```python
from build123d import *

# Parameters (mm, degrees)
SKETCH1_R           = 125
SKETCH1_R_2         = 2.5
BOSS_EXTRUDE1_DEPTH = 4


with BuildPart() as part:
    # Sketch1 → Boss-Extrude1 (new body)
    with BuildSketch(Plane(origin=(0, 0, 0), x_dir=(1, 0, 0), z_dir=(0, 1, 0))):
        Circle(SKETCH1_R)
        with Locations((-115, 0)):
            Circle(SKETCH1_R_2, mode=Mode.SUBTRACT)
        with Locations((-99.592921435, 57.5)):
            Circle(SKETCH1_R_2, mode=Mode.SUBTRACT)
        with Locations((-57.5, 99.592921435)):
            Circle(SKETCH1_R_2, mode=Mode.SUBTRACT)
        with Locations((0, 115)):
            Circle(SKETCH1_R_2, mode=Mode.SUBTRACT)
        with Locations((57.5, 99.592921435)):
            Circle(SKETCH1_R_2, mode=Mode.SUBTRACT)
        with Locations((99.592921435, 57.5)):
            Circle(SKETCH1_R_2, mode=Mode.SUBTRACT)
        with Locations((115, 0)):
            Circle(SKETCH1_R_2, mode=Mode.SUBTRACT)
        with Locations((99.592921435, -57.5)):
            Circle(SKETCH1_R_2, mode=Mode.SUBTRACT)
        with Locations((57.5, -99.592921435)):
            Circle(SKETCH1_R_2, mode=Mode.SUBTRACT)
        with Locations((0, -115)):
            Circle(SKETCH1_R_2, mode=Mode.SUBTRACT)
        with Locations((-57.5, -99.592921435)):
            Circle(SKETCH1_R_2, mode=Mode.SUBTRACT)
        with Locations((-99.592921435, -57.5)):
            Circle(SKETCH1_R_2, mode=Mode.SUBTRACT)
        with BuildLine():
            Line((-89.732773716, 28.184928973), (-62.744806129, 20.953524853))
            ThreePointArc((-62.744806129, 20.953524853), (-59.916379005, 16.054545368), (-64.81535849, 13.226118243))
            Line((-64.81535849, 13.226118243), (-91.803326077, 20.457522363))
            ThreePointArc((-91.803326077, 20.457522363), (-94.631753202, 25.356501849), (-89.732773716, 28.184928973))
        make_face(mode=Mode.SUBTRACT)
        with BuildLine():
            Line((-93.131960654, 17.723307294), (-66.143993068, 10.491903174))
            ThreePointArc((-66.143993068, 10.491903174), (-63.315565943, 5.592923688), (-68.214545428, 2.764496564))
            Line((-68.214545428, 2.764496564), (-95.202513015, 9.995900684))
            ThreePointArc((-95.202513015, 9.995900684), (-98.03094014, 14.894880169), (-93.131960654, 17.723307294))
        make_face(mode=Mode.SUBTRACT)
        with BuildLine():
            Line((-96.531147592, 7.261685615), (-69.543180006, 0.030281495))
            ThreePointArc((-69.543180006, 0.030281495), (-66.714752881, -4.868697991), (-71.613732367, -7.697125116))
            Line((-71.613732367, -7.697125116), (-98.601699953, -0.465720995))
            ThreePointArc((-98.601699953, -0.465720995), (-101.430127078, 4.43325849), (-96.531147592, 7.261685615))
        make_face(mode=Mode.SUBTRACT)
        with BuildLine():
            Line((-99.93033453, -3.199936064), (-72.942366944, -10.431340184))
            ThreePointArc((-72.942366944, -10.431340184), (-70.113939819, -15.33031967), (-75.012919305, -18.158746795))
            Line((-75.012919305, -18.158746795), (-102.000886891, -10.927342675))
            ThreePointArc((-102.000886891, -10.927342675), (-104.829314016, -6.028363189), (-99.93033453, -3.199936064))
        make_face(mode=Mode.SUBTRACT)
        with BuildLine():
            Line((91.803326077, -20.457522363), (64.81535849, -13.226118243))
            ThreePointArc((64.81535849, -13.226118243), (59.916379005, -16.054545368), (62.744806129, -20.953524853))
            Line((62.744806129, -20.953524853), (89.732773716, -28.184928973))
            ThreePointArc((89.732773716, -28.184928973), (94.631753202, -25.356501849), (91.803326077, -20.457522363))
        make_face(mode=Mode.SUBTRACT)
        with BuildLine():
            Line((89.516297478, -31.217145971), (62.528329891, -23.985741851))
            ThreePointArc((62.528329891, -23.985741851), (57.629350406, -26.814168976), (60.45777753, -31.713148461))
            Line((60.45777753, -31.713148461), (87.445745117, -38.944552582))
            ThreePointArc((87.445745117, -38.944552582), (92.344724603, -36.116125457), (89.516297478, -31.217145971))
        make_face(mode=Mode.SUBTRACT)
        with BuildLine():
            Line((87.229268879, -41.976769579), (60.241301292, -34.745365459))
            ThreePointArc((60.241301292, -34.745365459), (55.342321807, -37.573792584), (58.170748931, -42.472772069))
            Line((58.170748931, -42.472772069), (85.158716518, -49.70417619))
            ThreePointArc((85.158716518, -49.70417619), (90.057696004, -46.875749065), (87.229268879, -41.976769579))
        make_face(mode=Mode.SUBTRACT)
        with BuildLine():
            Line((84.94224028, -52.736393187), (57.954272693, -45.504989067))
            ThreePointArc((57.954272693, -45.504989067), (53.055293208, -48.333416192), (55.883720332, -53.232395677))
            Line((55.883720332, -53.232395677), (82.871687919, -60.463799798))
            ThreePointArc((82.871687919, -60.463799798), (87.770667405, -57.635372673), (84.94224028, -52.736393187))
        make_face(mode=Mode.SUBTRACT)
        with BuildLine():
            Line((14.021652384, 104.900536337), (41.00961997, 97.669132217))
            ThreePointArc((41.00961997, 97.669132217), (43.838047095, 92.770152731), (38.939067609, 89.941725607))
            Line((38.939067609, 89.941725607), (11.951100023, 97.173129727))
            ThreePointArc((11.951100023, 97.173129727), (9.122672898, 102.072109212), (14.021652384, 104.900536337))
        make_face(mode=Mode.SUBTRACT)
        with BuildLine():
            Line((10.622465446, 94.438914658), (37.610433032, 87.207510538))
            ThreePointArc((37.610433032, 87.207510538), (40.438860157, 82.308531052), (35.539880671, 79.480103927))
            Line((35.539880671, 79.480103927), (8.551913085, 86.711508048))
            ThreePointArc((8.551913085, 86.711508048), (5.72348596, 91.610487533), (10.622465446, 94.438914658))
        make_face(mode=Mode.SUBTRACT)
        with BuildLine():
            Line((7.223278507, 83.977292979), (34.211246094, 76.745888859))
            ThreePointArc((34.211246094, 76.745888859), (37.039673219, 71.846909373), (32.140693733, 69.018482248))
            Line((32.140693733, 69.018482248), (5.152726147, 76.249886368))
            ThreePointArc((5.152726147, 76.249886368), (2.324299022, 81.148865854), (7.223278507, 83.977292979))
        make_face(mode=Mode.SUBTRACT)
        with BuildLine():
            Line((3.824091569, 73.515671299), (30.812059156, 66.284267179))
            ThreePointArc((30.812059156, 66.284267179), (33.640486281, 61.385287694), (28.741506795, 58.556860569))
            Line((28.741506795, 58.556860569), (1.753539208, 65.788264689))
            ThreePointArc((1.753539208, 65.788264689), (-1.074887916, 70.687244175), (3.824091569, 73.515671299))
        make_face(mode=Mode.SUBTRACT)
    extrude(amount=BOSS_EXTRUDE1_DEPTH)


solid = part.part
```
Geometry: final body of the model. Coordinates: model frame, mm. Round coordinates to 2 decimals unless told otherwise and drop trailing zeros. Order: outer loops, then holes, each group sorted by start corner. A loop starts at its lowest first (then second) coordinate and runs counter-clockwise, first axis right, second up. Notation, with made-up numbers: (25.5, -14.75) -> (44.5, -14.75) arc R17 cw to (44.5, -9.75) -> close; hole circle Ø6 at (36, -5.75). An arc over 180 degrees is marked (long way). Use one line per item in the form item = value.
(1) Section A-A on x = 77.5. Return loops of the section in (y, z), and give its area (3 significant figures).
Results list:
outline = (0, -98.08) -> (4, -98.08) -> (4, 16.62) -> (0, 16.62) -> close; (0, 24.91) -> (4, 24.91) -> (4, 28) -> (0, 28) -> close; (0, 36.28) -> (4, 36.28) -> (4, 39.37) -> (0, 39.37) -> close; (0, 47.65) -> (4, 47.65) -> (4, 50.74) -> (0, 50.74) -> close; (0, 59.02) -> (4, 59.02) -> (4, 98.08) -> (0, 98.08) -> close
area = 652 mm^2
(2) Section D-D on z = 66. Return loops of the section in (x, y), and give its area (3 significant figures).
Results list:
outline = (-106.16, 0) -> (106.16, 0) -> (106.16, 4) -> (-106.16, 4) -> close
area = 849 mm^2
(3) Draft query along Z for faces 1 (the face through (-124.88, 1.97, -5.5)), 2 (the face through (-2, 4, -2)), 3 (the face through (-81.52, 1.97, -6.33)). Return one class per face: pulls with the +Z half, pulls with the -Z half, needs draft (parallel to the pull), parting line crosses it, or undercut.
Results list:
face_1 = parting line crosses it
face_2 = needs draft
face_3 = undercut
(4) Ray query, probe 1 along Z at (x, y) = (99.5, 0.45); probe 2 along Z at (x, y) = (-90, 0.7); probe 3 along X at (y, z) = (3, 115). Return the intervals inside material, ascending. Write a range as [from, to].
Results list:
probe_1 = [-75.66, -60], [-55, 55], [60, 75.66]
probe_2 = [-86.75, -28.25], [-19.97, -16.88], [-8.6, -5.51], [2.77, 5.86], [14.14, 86.75]
probe_3 = [-48.99, -2.5], [2.5, 48.99]
(5) Section C-C on y = 1.6. Count the separate pieces of the cut face and the enclosed holes in it, and give its area (3 significant figures).
Results list:
separate_pieces = 1
enclosed_holes = 24
area = 45,600 mm^2
(6) First-contact query: pin 1 Ø1.5 at (y, z) = (1.5, 74) entering from +X; pin 2 Ø4 at (x, z) = (57.5, 99.59) entering from -Y. Flat tips, straight axial feed; report the tip coordinate or a pass-through.
Results list:
pin_1 = 101.29
pin_2 = through
(7) Section B-B on x = -45. Return loops of the section in (y, z), and give its area (3 significant figures).
Results list:
outline = (0, -116.62) -> (4, -116.62) -> (4, 116.62) -> (0, 116.62) -> close
area = 933 mm^2
